Check sheet for the modelled part. Datum: model origin and axes. Units: mm. Face numbers are marked on the shaded views. Round coordinates to 2 decimals unless told otherwise and drop trailing zeros. Write each loop counter-clockwise with the first axis right and the second up, starting at its lowest first coordinate (ties: lowest second). Pieces come first, ordered by that corner, then holes. Notation, with made-up numbers: (82, -37.5) -> (94, -37.5) arc R14 cw to (94, -26.5) -> close; hole circle Ø6 at (4, 34). An arc over 180 degrees is marked (long way). Use one line per item in the form item = value. Start each with the question number.
Autodesk Inventor part; units mm, degrees
ref_plane "YZ Plane" through (0, 0, 0) normal (1, 0, 0) x (0, 1, 0)
ref_plane "XZ Plane" through (0, 0, 0) normal (0, 1, 0) x (-1, 0, 0)
ref_plane "XY Plane" through (0, 0, 0) normal (0, 0, 1) x (1, 0, 0)
sketch "Sketch1" plane through (0, 0, 0) normal (0, 0, 1) x (1, 0, 0)
  line L0 (0, 0) -> (50.8, 0)
  line L1 (0, 0) -> (0, 50.8)
  line L2 (6.35, 50.8) -> (6.35, 6.35)
  line L3 (6.35, 6.35) -> (50.8, 6.35)
  line L4 (0, 50.8) -> (6.35, 50.8)
  line L5 (50.8, 6.35) -> (50.8, 0)
  dimension "d0" = 50.8
  dimension "d1" = 50.8
  dimension "d2" = 6.35
extrude "Extrusion1" add sketch "Sketch1" along normal mid plane 110
sketch "Sketch9" plane through (6.35, 6.35, 55) normal (1, 0, 0) x (0, 0, -1)
  line L0 (30, 44.45) -> (80, 44.45)
  line L1 (80, 44.45) -> (80, 8.45)
  line L2 (80, 8.45) -> (30, 8.45)
  line L3 (30, 8.45) -> (30, 44.45)
  line L4 (110, 44.45) -> (0, 44.45)
  point P0 (55, -6.35)
  point P1 (55, 44.45)
  dimension "d140" = 50
  dimension "d141" = 36
extrude "Extrusion8" cut sketch "Sketch9" against normal through all
sketch "Sketch8" plane through (6.35, 6.35, 55) normal (1, 0, 0) x (0, 0, -1)
  circle A0 centre (7, 38.45) radius 4
  circle A1 centre (21, 38.45) radius 4
  line L0 (0, 0) -> (0, 44.45) construction
  line L1 (110, 44.45) -> (0, 44.45) construction
  circle A2 centre (7, 24.45) radius 4
  circle A3 centre (21, 24.45) radius 4
  line L2 (55, 44.45) -> (55, 8.45) construction
  line L3 (30, 8.45) -> (80, 8.45) construction
  circle A4 centre (103, 38.45) radius 4
  circle A5 centre (89, 38.45) radius 4
  circle A6 centre (103, 24.45) radius 4
  circle A7 centre (89, 24.45) radius 4
  circle A8 centre (7, 8.45) radius 3
  circle A9 centre (21, 8.45) radius 3
  circle A10 centre (103, 8.45) radius 3
  circle A11 centre (89, 8.45) radius 3
  point P0 (55, -6.35)
  dimension "d135" = 8
  dimension "d136" = 8
  dimension "d137" = 7
  dimension "d138" = 6
  dimension "d139" = 14
  dimension "d146" = 14
  dimension "d160" = 6
  dimension "d161" = 16
  dimension "d162" = 6
extrude "Extrusion9" cut sketch "Sketch8" against normal through all
hole "Hole2" at (6.35, 14.8, 48) at (6.35, 14.8, 34) at (6.35, 14.8, -34) at (6.35, 14.8, -48) direction (-1, 0, 0) diameter 6 end through all countersink diameter 12 countersink angle 90
sketch "Sketch10" plane through (6.35, 6.35, 55) normal (0, 1, 0) x (1, 0, 0)
  circle A0 centre (38.45, 6) radius 4
  line L0 (44.45, 0) -> (0, 0) construction
  line L1 (44.45, 110) -> (44.45, 0) construction
  circle A1 centre (38.45, 20) radius 4
  circle A2 centre (24.45, 6) radius 4
  circle A3 centre (24.45, 20) radius 4
  circle A4 centre (8.45, 6) radius 3
  circle A5 centre (8.45, 20) radius 3
  line L2 (0, 110) -> (0, 0) construction
  line L3 (0, 55) -> (44.45, 55) construction
  circle A6 centre (38.45, 104) radius 4
  circle A7 centre (38.45, 90) radius 4
  circle A8 centre (24.45, 104) radius 4
  circle A9 centre (24.45, 90) radius 4
  circle A10 centre (8.45, 104) radius 3
  circle A11 centre (8.45, 90) radius 3
  point P0 (-6.35, 55)
  dimension "d170" = 8
  dimension "d171" = 6
  dimension "d172" = 6
  dimension "d173" = 8
  dimension "d174" = 14
  dimension "d177" = 14
  dimension "d182" = 6
  dimension "d183" = 16
  dimension "d184" = 6
extrude "Extrusion10" cut sketch "Sketch10" against normal through all
hole "Hole3" at (14.8, 6.35, 49) at (14.8, 6.35, 35) at (14.8, 6.35, -35) at (14.8, 6.35, -49) direction (0, -1, 0) diameter 6 end through all countersink diameter 12 countersink angle 90
sketch "Sketch11" plane through (6.35, 6.35, 55) normal (0, 1, 0) x (1, 0, 0)
  line L0 (44.45, 110) -> (44.45, 0) construction
  line L1 (44.45, 80) -> (8.45, 80)
  line L2 (8.45, 80) -> (8.45, 30)
  line L3 (8.45, 30) -> (44.45, 30)
  line L4 (44.45, 30) -> (44.45, 80)
  line L5 (0, 80) -> (0, 30) construction
  point P0 (-6.35, 55)
  dimension "d194" = 36
extrude "Extrusion11" cut sketch "Sketch11" against normal through all
chamfer "Chamfer1" distance 4 angle 45 2 edges at (50.8, 3.175, 25) (50.8, 3.175, -25)
fillet "Fillet1" radius 4 2 edges at (14.8, 3.175, -25) (14.8, 3.175, 25)
fillet "Fillet2" radius 4 2 edges at (3.175, 14.8, 25) (3.175, 14.8, -25)
properties part number "LongL-Bracket"
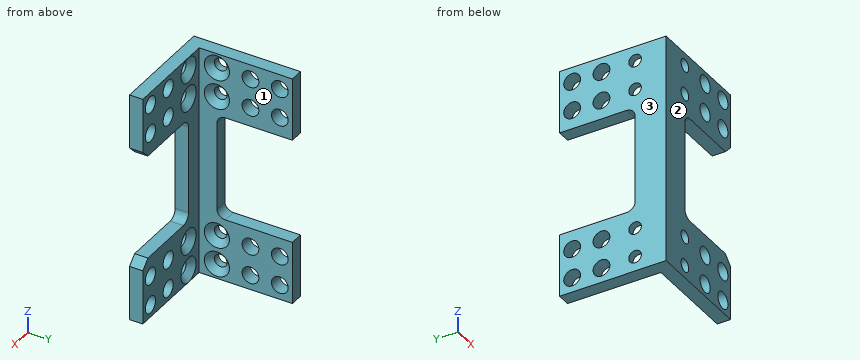
1. Sectioned sample at A-A (x = 30.8). Enter the section's corners in (y, z), and give its area (3 significant figures).
2. Depth check by flat-ended pin: pin 1 (7 mm diameter, centred on y = 14.8, z = -48, fed in from +X); pin 2 (6 mm diameter, centred on y = 9, z = 7, fed in from -X); pin 3 (5 mm diameter, centred on y = 14.8, z = -34, fed in from -X); pin 4 (10.5 mm diameter, centred on y = 44.8, z = 48, fed in from +X). Enter the tip coordinate at first touch or a pass-through.
3. Mould release check, pull along X, two halves, no side actions. Record for the marked faces 1, 2 and 3: +X half, -X half, draft (parallel to the pull), parting line (faces both ways), or undercut.
4. Scan lines: probe 1 along X at (y, z) = (2.75, 35); probe 2 along Z at (x, y) = (44.8, 2.25). Record each from-to range of solid material in increasing order.
5. Sectioned sample at D-D (z = -49). Give the number of separate pieces and of enclosed holes in the cut face, and give its area (3 significant figures).
6. Sectioned sample at C-C (x = 25). Enter the section's corners in (y, z).
7. Sectioned sample at B-B (y = 30.8). Enter the section's corners in (x, z), and give its area (3 significant figures).
Returned:
q1.outline = (0, -55) -> (6.35, -55) -> (6.35, -53) -> (0, -53) -> close; (0, -45) -> (6.35, -45) -> (6.35, -39) -> (0, -39) -> close; (0, -31) -> (6.35, -31) -> (6.35, -25) -> (0, -25) -> close; (0, 25) -> (6.35, 25) -> (6.35, 31) -> (0, 31) -> close; (0, 39) -> (6.35, 39) -> (6.35, 45) -> (0, 45) -> close; (0, 53) -> (6.35, 53) -> (6.35, 55) -> (0, 55) -> close
q1.area = 178 mm^2
q2.pin_1 = 3.85
q2.pin_2 = 0
q2.pin_3 = through
q2.pin_4 = 6.35
q3.face_1 = +X half
q3.face_2 = draft
q3.face_3 = -X half
q4.probe_1 = 0 to 11.8, 17.8 to 26.8, 34.8 to 40.8, 48.8 to 50.8
q4.probe_2 = -55 to -53, -45 to -39, -31 to -25, 25 to 31, 39 to 45, 53 to 55
q5.separate_pieces = 7
q5.enclosed_holes = 0
q5.area = 313 mm^2
q6.outline = (0, -55) -> (6.35, -55) -> (6.35, -25) -> (0, -25) -> close; (0, 25) -> (6.35, 25) -> (6.35, 55) -> (0, 55) -> close
q7.outline = (0, -55) -> (6.35, -55) -> (6.35, -52) -> (0, -52) -> close; (0, -44) -> (6.35, -44) -> (6.35, -38) -> (0, -38) -> close; (0, -30) -> (6.35, -30) -> (6.35, -25) -> (0, -25) -> close; (0, 25) -> (6.35, 25) -> (6.35, 30) -> (0, 30) -> close; (0, 38) -> (6.35, 38) -> (6.35, 44) -> (0, 44) -> close; (0, 52) -> (6.35, 52) -> (6.35, 55) -> (0, 55) -> close
q7.area = 178 mm^2
